from build123d import *

# Parameters (mm, degrees)
BOSS_EXTRUDE1_DEPTH = 30
SKETCH2_R           = 25
BOSS_EXTRUDE2_DEPTH = 90
SKETCH3_R           = 12.5
CUT_EXTRUDE1_DEPTH  = 31


with BuildPart() as part:
    # Sketch1 → Boss-Extrude1 (new body)
    with BuildSketch(Plane(origin=(0, 0, 0), x_dir=(1, 0, 0), z_dir=(0, 1, 0))):
        with BuildLine():
            Line((115, -75), (-115, -75))
            ThreePointArc((-115, -75), (-122.071067812, -72.071067812), (-125, -65))
            Line((-125, -65), (-125, 65))
            ThreePointArc((-125, 65), (-122.071067812, 72.071067812), (-115, 75))
            Line((-115, 75), (115, 75))
            ThreePointArc((115, 75), (122.071067812, 72.071067812), (125, 65))
            Line((125, 65), (125, -65))
            ThreePointArc((125, -65), (122.071067812, -72.071067812), (115, -75))
        make_face()
    extrude(amount=BOSS_EXTRUDE1_DEPTH)

    # Sketch2 → Boss-Extrude2 (add)
    with BuildSketch(Plane(origin=(0, 30, 0), x_dir=(1, 0, 0), z_dir=(0, 1, 0))):
        with Locations((0, 25)):
            Circle(SKETCH2_R)
    extrude(amount=BOSS_EXTRUDE2_DEPTH)

    # Sketch3 → Cut-Extrude1 (cut, through all)
    with BuildSketch(Plane(origin=(0, 30, 0), x_dir=(1, 0, 0), z_dir=(0, 1, 0))):
        with Locations((-95, 45)):
            Circle(SKETCH3_R)
        with Locations((95, 45)):
            Circle(SKETCH3_R)
        with Locations((95, -45)):
            Circle(SKETCH3_R)
        with Locations((-95, -45)):
            Circle(SKETCH3_R)
    extrude(amount=-CUT_EXTRUDE1_DEPTH, mode=Mode.SUBTRACT)


solid = part.part
Verification items for the finished model (mm, model axes). A direction names the side the tool comes from. Coordinates: 2 decimals unless noted, no trailing zeros. Write each loop counter-clockwise with the first axis right and the second up, starting at its lowest first coordinate (ties: lowest second). Pieces come first, ordered by that corner, then holes. Notation, with made-up numbers: M 29.25,85.25 L 85.25,85.25 A25 cw 85.25,103.25 Z; hole C -4,-39.5 d3. An arc over 180 degrees is marked long. Use CSV: the item, a comma, the result in double quotes.
Q1. Mould release check, pull along X, two halves, no side actions. Record for faces 1 (the cylindrical face through (-83.453, 15.21, -40.212)), 2 (the flat face through (-125, 15, 1)), 3 (the cylindrical face through (121.99, 14.79, -72.15)): pulls with the +X half, pulls with the -X half, needs draft (parallel to the pull), parting line crosses it, or undercut.
Computed values:
face 1,"undercut"
face 2,"pulls with the -X half"
face 3,"pulls with the +X half"
Q2. Go/stop test with flat-tipped pins: P1, Ø1, axis at x = 4.5, z = 3.5, coming from the +Y side; P2, Ø3, axis at x = 18, y = 100.5, coming from the +Z side. Record where each tip stops, or that it passes through.
Computed values:
P1,"y = 30"
P2,"z = -6.22"
Q3. Section check D-D, the plane y = 21. Enter the section's corners in (x, z), and give its area (3 significant figures).
Computed values:
outline,"M -125,-65 A10 ccw -115,-75 L 115,-75 A10 ccw 125,-65 L 125,65 A10 ccw 115,75 L -115,75 A10 ccw -125,65 Z; hole C -95,-45 d25; hole C -95,45 d25; hole C 95,-45 d25; hole C 95,45 d25"
area,"35,500 mm²"
Q4. Section check C-C, the plane z = -25. Enter the section's corners in (x, y).
Computed values:
outline,"M -125,0 L 125,0 L 125,30 L 25,30 L 25,120 L -25,120 L -25,30 L -125,30 Z"
Q5. Section check A-A, the plane x = -95. Enter the section's corners in (y, z), and give its area (3 significant figures).
Computed values:
outline,"M 0,-75 L 30,-75 L 30,-57.5 L 0,-57.5 Z; M 0,-32.5 L 30,-32.5 L 30,32.5 L 0,32.5 Z; M 0,57.5 L 30,57.5 L 30,75 L 0,75 Z"
area,"3,000 mm²"
Q6. Section check B-B, the plane z = 45. Enter the section's corners in (x, y).
Computed values:
outline,"M -125,0 L -107.5,0 L -107.5,30 L -125,30 Z; M -82.5,0 L 82.5,0 L 82.5,30 L -82.5,30 Z; M 107.5,0 L 125,0 L 125,30 L 107.5,30 Z"
Q7. Thickness scan on line 1 along X through (y, z) = (12, -45); line 2 along Z through (x, y) = (-97, 10); line 3 along Y through (x, z) = (83, -10). Record the ranges inside material, lowest first. Write a range as [from, to].
Computed values:
line 1,"[-125, -107.5], [-82.5, 82.5], [107.5, 125]"
line 2,"[-75, -57.34], [-32.66, 32.66], [57.34, 75]"
line 3,"[0, 30]"
Q8. Set-up check for faces 4 (the flat face through (125, 15, -1)), 5 (the cylindrical face through (11.5, 74.4, -2.8)): record each of +Z, -Z, +X, -X, +Y, -Y from which the full face is reachable in a straight line by a thin tool's end or side.
Computed values:
face 4,"+Z, -Z, +X, +Y, -Y"
face 5,"+Y"
